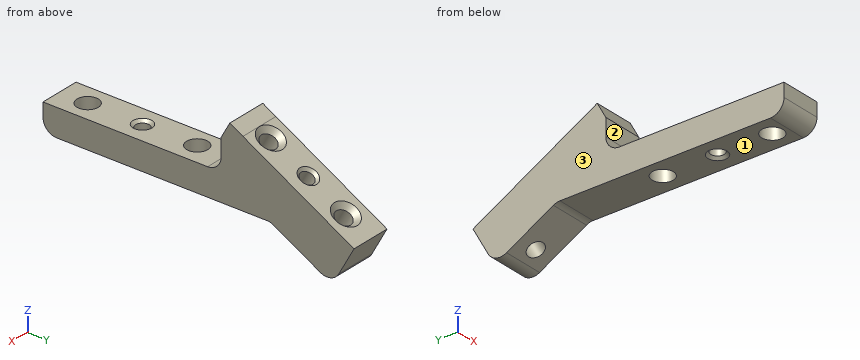
from build123d import *

# Parameters (mm, degrees)
BOSS_EXTRUDE1_DEPTH                    = 9.525
SKETCH2_W                              = 9.525
SKETCH2_H                              = 29.633356585
BOSS_EXTRUDE2_DEPTH                    = 10.5
BOSS_EXTRUDE3_DEPTH                    = 9.525
CUT_EXTRUDE1_DEPTH                     = 9.525
FILLET1_R                              = 3.175
F_10_24_TAPPED_HOLE1_D                 = 3.7973
F_10_24_TAPPED_HOLE1_DEPTH             = 12.83
F_10_24_TAPPED_HOLE1_CSINK_D           = 6.096
F_10_24_TAPPED_HOLE1_CSINK_ANGLE       = 90
F_10_24_TAPPED_HOLE1_TIP               = 1.140824014
F_1_8_0_125_DIAMETER_HOLE1_D           = 3.175
F_1_8_0_125_DIAMETER_HOLE1_DEPTH       = 8
F_1_8_0_125_DIAMETER_HOLE1_CSINK_D     = 4.445
F_1_8_0_125_DIAMETER_HOLE1_CSINK_ANGLE = 90
F_1_8_0_125_DIAMETER_HOLE1_TIP         = 0.953866233
F_10_CLEARANCE_HOLE1_D                 = 4.9784


with BuildPart() as part:
    # Sketch1 → Boss-Extrude1 (new body)
    with BuildSketch(Plane(origin=(0, 0, 0), x_dir=(0, 0, -1), z_dir=(1, 0, 0))):
        Polygon((0, 0), (13.510509947, 24.524806237), (7.948634247, 27.588796886), (-6.35, 1.633356585), (-6.35, -40), (0, -40), align=None)
    extrude(amount=BOSS_EXTRUDE1_DEPTH)

    # Sketch2 → Boss-Extrude2 (add)
    with BuildSketch(Plane(origin=(0, 3.063990649, 5.5618757), x_dir=(1, 0, 0), z_dir=(0, 0.482518212, 0.875885937))):
        with Locations((4.7625, 13.183321707)):
            Rectangle(SKETCH2_W, SKETCH2_H)
    extrude(amount=BOSS_EXTRUDE2_DEPTH)

    # Sketch3 → Boss-Extrude3 (add)
    with BuildSketch(Plane.ZY):
        Polygon((15.546802339, 6.699797816), (6.35, 1.633356585), (13.599802436, 1.633356585), (17.234729075, 3.635807167), align=None)
    extrude(amount=-BOSS_EXTRUDE3_DEPTH)

    # Sketch4 → Cut-Extrude1 (cut)
    with BuildSketch(Plane(origin=(9.525, 0, 0), x_dir=(0, 0, -1), z_dir=(1, 0, 0))):
        Polygon((13.510509947, 24.524806237), (7.948634247, 27.588796886), (0, 13.160125021), (0, 0), align=None)
    extrude(amount=-CUT_EXTRUDE1_DEPTH, mode=Mode.SUBTRACT)

    # Fillet1
    fillet1_edges = [part.edges().sort_by_distance(p)[0] for p in [
        (4.7625, -40, 0),
        (4.7625, 1.633356585, 6.35),
        (4.7625, 27.588796886, -7.948634247),
        (4.7625, 13.160125021, 0),
    ]]
    fillet(fillet1_edges, radius=FILLET1_R)

    # #10-24 Tapped Hole1
    with Locations(Plane(origin=(0, 8.130431879, 14.758678039), x_dir=(1, 0, 0), z_dir=(0, 0.482518212, 0.875885937))):
        with Locations((4.7625, 21.434240851), (4.7625, 1.434240851)):
            CounterSinkHole(F_10_24_TAPPED_HOLE1_D / 2, F_10_24_TAPPED_HOLE1_CSINK_D / 2, depth=F_10_24_TAPPED_HOLE1_DEPTH, counter_sink_angle=F_10_24_TAPPED_HOLE1_CSINK_ANGLE)
            with Locations((0, 0, -(F_10_24_TAPPED_HOLE1_DEPTH + F_10_24_TAPPED_HOLE1_TIP / 2))):  # 118° drill point
                Cone(0, F_10_24_TAPPED_HOLE1_D / 2, F_10_24_TAPPED_HOLE1_TIP, mode=Mode.SUBTRACT)

    # 1/8 (0.125) Diameter Hole1
    with Locations(Plane(origin=(0, 8.130431879, 14.758678039), x_dir=(1, 0, 0), z_dir=(0, 0.482518212, 0.875885937))):
        with Locations((4.7625, 11.434240851)):
            CounterSinkHole(F_1_8_0_125_DIAMETER_HOLE1_D / 2, F_1_8_0_125_DIAMETER_HOLE1_CSINK_D / 2, depth=F_1_8_0_125_DIAMETER_HOLE1_DEPTH, counter_sink_angle=F_1_8_0_125_DIAMETER_HOLE1_CSINK_ANGLE)
            with Locations((0, 0, -(F_1_8_0_125_DIAMETER_HOLE1_DEPTH + F_1_8_0_125_DIAMETER_HOLE1_TIP / 2))):  # 118° drill point
                Cone(0, F_1_8_0_125_DIAMETER_HOLE1_D / 2, F_1_8_0_125_DIAMETER_HOLE1_TIP, mode=Mode.SUBTRACT)

    # #10 Clearance Hole1 (through all)
    with Locations(Plane.XY.offset(6.35)):
        with Locations((4.7625, -33.418643415), (4.519767079, -8.018643415)):
            Hole(F_10_CLEARANCE_HOLE1_D / 2)

    # Sketch12 → 1/8 (0.125) Diameter Hole2 (revolve, cut)
    with BuildSketch(Plane(origin=(4.641133539, -20.718643415, 6.35), x_dir=(0, -1, 0), z_dir=(1, 0, 0))):
        Polygon((0, 0), (0, 6.35), (2.2225, 6.35), (1.5875, 5.715), (1.5875, 0.635), (2.2225, 0), align=None)
    revolve(axis=Axis((4.641133539, -20.718643415, 12.7), (0, 0, -1)), mode=Mode.SUBTRACT)


solid = part.part
Geometry check sheet. Reference: the model listing, model coordinates, mm. Face numbers are marked on the shaded views. A direction names the side the tool comes from. Round coordinates to 2 decimals unless told otherwise and drop trailing zeros. Loops run counter-clockwise (first coordinate to the right, second up) from the corner with the lowest first, then second, coordinate; pieces in that order, holes last. Notation, with made-up numbers: (1.25, 39.25) - (33.25, 39.25) arc R15 ccw to (33.25, 45.25) - close; hole circle Ø6 at (26.5, -10). An arc over 180 degrees is marked (long way). One line per question, with ' | ' between items. Start each with the question number.
1. Tool access check on the marked faces 1, 2 and 3. Record the directions out of +Z, -Z, +X, -X, +Y, -Y that give a thin tool (end or side, any length) a straight path to the whole face; none if there is none.
2. Depth check by flat-ended pin: pin 1 (1.5 mm diameter, centred on x = 2, y = 2.5, fed in from -Z); pin 2 (1.9 mm diameter, centred on x = 4.64, y = -20.72, fed in from +Z); pin 3 (1 mm diameter, centred on x = 1.5, z = -0.5, fed in from +Y); pin 4 (5 mm diameter, centred on x = 3, y = -25, fed in from +Z). Enter the tip coordinate at first touch or a pass-through.
3. Cross-section at A-A on y = -3. Record the cut outline in (x, z) (3 decimals), then the cut area to 3 significant figures.
4. Scan lines: line 1 (Y direction, x = 4.25, z = 4.5); line 2 (Y direction, x = 9.25, z = 15.25); line 3 (Z direction, x = 7.75, y = -18). Record each from-to range of solid material in increasing order. Write a range as [from, to].
Taken from the geometry:
1) face 1: -Z, +X, -X, -Y | face 2: +Z, +X, -X, -Y | face 3: +Z, -Z, -X, +Y, -Y
2) pin 1: z = 0 | pin 2: through | pin 3: y = 31.97 | pin 4: z = 6.35
3) outline: (0, 0) - (9.525, 0) - (9.525, 6.35) - (0, 6.35) - close | area: 60.5 mm²
4) line 1: [-40, -35.85], [-30.98, -22.26], [-19.18, -10.49], [-5.54, 2.03], [6.2, 13.82], [17.25, 24.68] | line 2: [2.54, 7.24] | line 3: [0, 6.35]
